Source: three-view drawing plus pictorial views. Frame: mm from the lowest corner of the part. Give positions to 0.01 mm unless a question says otherwise; leave off trailing zeros. Write each loop counter-clockwise with the first axis right and the second up, starting at its lowest first coordinate (ties: lowest second). Pieces come first, ordered by that corner, then holes.
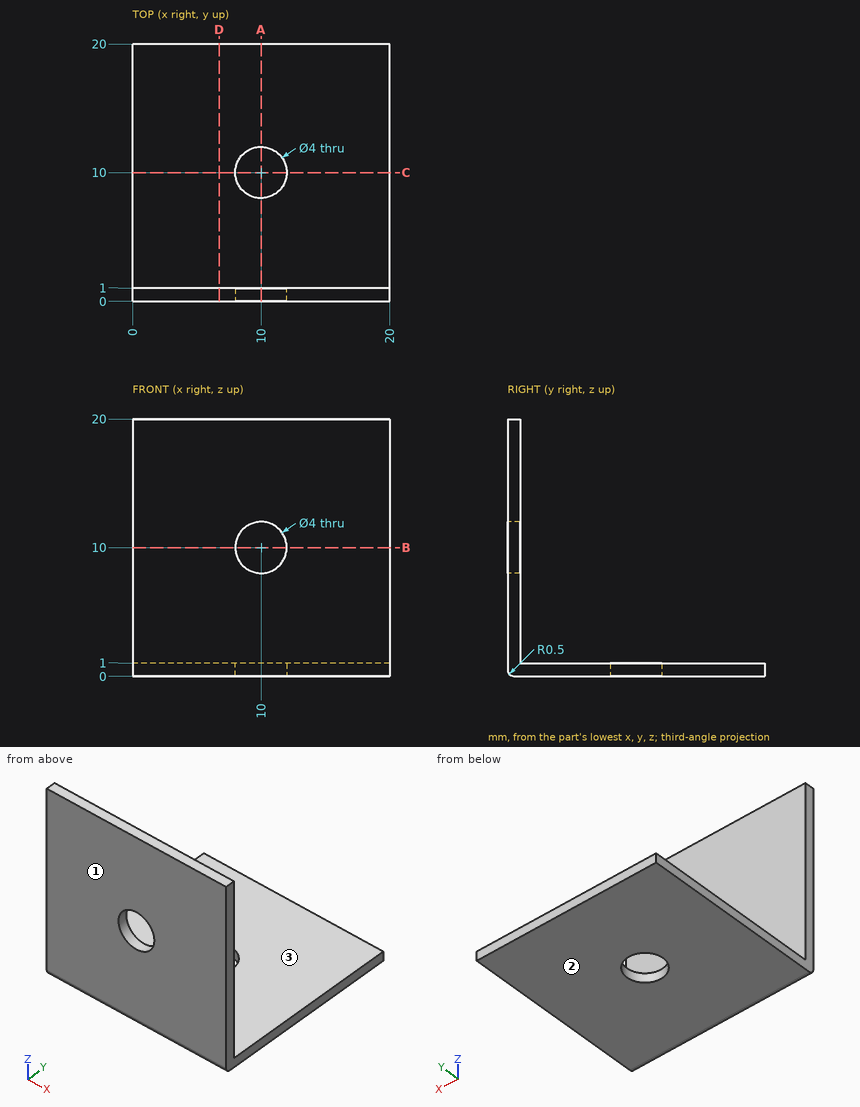
Q1. Pin query (flat end, axial travel): P1, Ø1.5, axis at x = 9, y = 8, coming from the +Z side; P2, Ø5, axis at x = 10, z = 10, coming from the -Y side; P3, Ø12, axis at x = 8, z = 17, coming from the +Y side. Return the tip coordinate at first contact, or that it passes through.
Filled sheet:
P1: stops at z = 1
P2: stops at y = 0
P3: stops at y = 1
Q2. Ray query, line 1 along Y through (x, z) = (1.5, 2.75); line 2 along Z through (x, y) = (10, 0.3). Return the intervals inside material, ascending.
Filled sheet:
line 1: y = 0 to 1
line 2: z = 0.04 to 8, 12 to 20
Q3. Pull-direction query (Z, two-part tool) for the marked faces 1, 2 and 3; classes: released by +Z, released by -Z, zero draft, split by the parting line, or undercut.
Filled sheet:
face 1: zero draft
face 2: released by -Z
face 3: released by +Z
Q4. Section D-D on x = 6.75. Output: boundary loops of the cut face in (y, z).
Filled sheet:
outline: (0, 0.5) arc R0.5 ccw to (0.5, 0) - (20, 0) - (20, 1) - (1, 1) - (1, 20) - (0, 20) - close
Q5. Section B-B on z = 10. Output: boundary loops of the cut face in (x, y).
Filled sheet:
outline: (0, 0) - (8, 0) - (8, 1) - (0, 1) - close; (12, 0) - (20, 0) - (20, 1) - (12, 1) - close
Q6. Section A-A on x = 10. Output: boundary loops of the cut face in (y, z).
Filled sheet:
outline: (0, 0.5) arc R0.5 ccw to (0.5, 0) - (8, 0) - (8, 1) - (1, 1) - (1, 8) - (0, 8) - close; (0, 12) - (1, 12) - (1, 20) - (0, 20) - close; (12, 0) - (20, 0) - (20, 1) - (12, 1) - close
